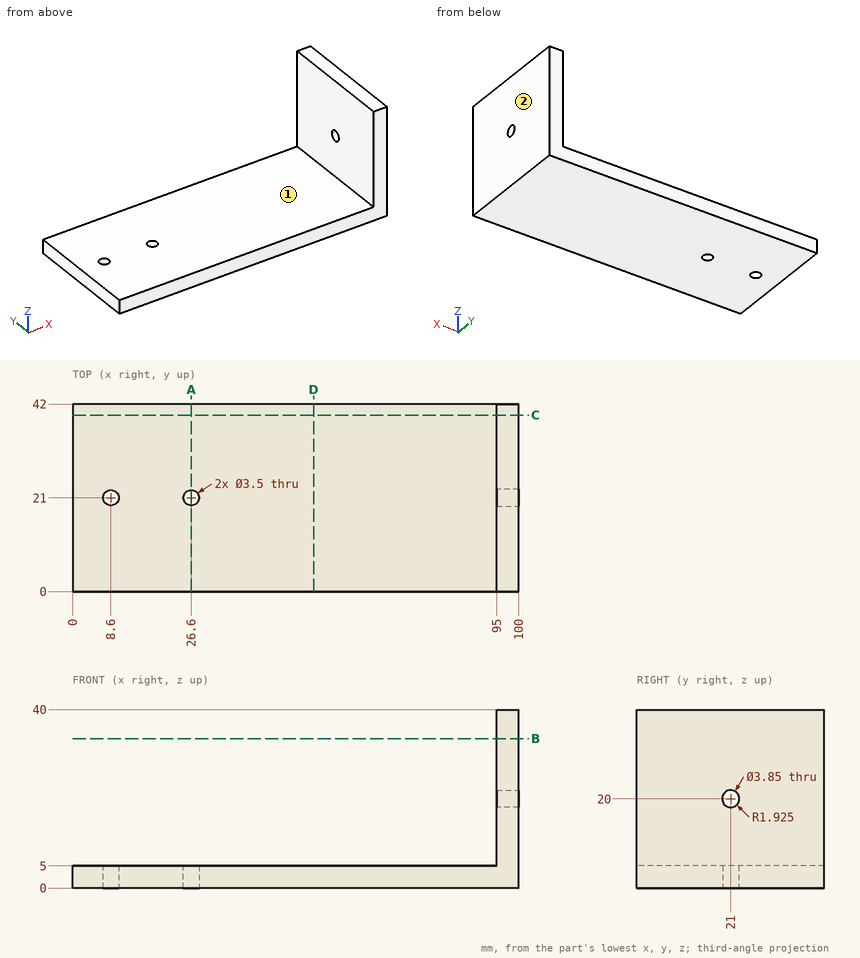
Geometry check sheet. Reference: drawing and pictorial views, mm from the part's lowest x, y, z. A direction names the side the tool comes from. Give positions to 0.01 mm unless a question says otherwise; leave off trailing zeros. Loops run counter-clockwise (first coordinate to the right, second up) from the corner with the lowest first, then second, coordinate; pieces in that order, holes last. Notation, with made-up numbers: M -14.75,4.25 L 14.25,4.25 A8 cw 14.25,12.25 Z; hole C -30.5,-13.5 d6. An arc over 180 degrees is marked long. Use a Markdown table: item, result. Add a question column.
Q1. Sectioned sample at A-A, the plane x = 26.6. Record the cut outline in (y, z).
Q2. Sectioned sample at B-B, the plane z = 33.5. Record the cut outline in (x, y), then the cut area to 3 significant figures.
Q3. Go/stop test with flat-tipped pins: pin 1 (5 mm diameter, centred on y = 20.5, z = 8.5, fed in from -X); pin 2 (2 mm diameter, centred on x = 65, y = 28.5, fed in from +Z); pin 3 (3.5 mm diameter, centred on y = 21, z = 20, fed in from +X). Record where each tip stops, or that it passes through.
Q4. Scan lines: line 1 along Z through (x, y) = (96.05, 21) (3 decimals); line 2 along X through (y, z) = (23, 27); line 3 along Y through (x, z) = (8.6, 2.7). Record each from-to range of solid material in increasing order. Write a range as [from, to].
Q5. Tool access check on the marked faces 1 and 2. Record the directions out of +Z, -Z, +X, -X, +Y, -Y that give a thin tool (end or side, any length) a straight path to the whole face; none if there is none.
Q6. Sectioned sample at D-D, the plane x = 54. Record the cut outline in (y, z).
Q7. Sectioned sample at C-C, the plane y = 39.5. Record the cut outline in (x, z).
Verdict:
| question | item | result |
|---|---|---|
| 1 | outline | M 0,0 L 19.25,0 L 19.25,5 L 0,5 Z; M 22.75,0 L 42,0 L 42,5 L 22.75,5 Z |
| 2 | outline | M 95,0 L 100,0 L 100,42 L 95,42 Z |
| 2 | area | 210 mm^2 |
| 3 | pin 1 | x = 95 |
| 3 | pin 2 | z = 5 |
| 3 | pin 3 | through |
| 4 | line 1 | [0, 18.075], [21.925, 40] |
| 4 | line 2 | [95, 100] |
| 4 | line 3 | [0, 19.25], [22.75, 42] |
| 5 | face 1 | +Z, -X, +Y, -Y |
| 5 | face 2 | +Z, -Z, +X, +Y, -Y |
| 6 | outline | M 0,0 L 42,0 L 42,5 L 0,5 Z |
| 7 | outline | M 0,0 L 100,0 L 100,40 L 95,40 L 95,5 L 0,5 Z |
